Read the model definition and answer for the solid it produces. Units are mm, in the model's axes. Face numbers are marked on the shaded views. A direction names the side the tool comes from. Round coordinates to 2 decimals unless told otherwise and drop trailing zeros. Loops run counter-clockwise (first coordinate to the right, second up) from the corner with the lowest first, then second, coordinate; pieces in that order, holes last. Notation, with made-up numbers: (-30.5, 74.25) -> (23.5, 74.25) arc R24 cw to (23.5, 89.25) -> close; hole circle Ø1 at (29.5, 61.5). An arc over 180 degrees is marked (long way). Put each result on its own line as item: value.
from build123d import *

# Parameters (mm, degrees)
BOSS_EXTRUDE1_DEPTH = 5
SKETCH2_R           = 5
CUT_EXTRUDE1_DEPTH  = 3.5
SKETCH3_R           = 1
CUT_EXTRUDE2_DEPTH  = 2
CHAMFER3_SIZE       = 1.5


with BuildPart() as part:
    # Sketch1 → Boss-Extrude1 (new body)
    with BuildSketch(Plane.XY):
        with BuildLine():
            Line((0, -6.5), (13.5, -6.5))
            Line((13.5, -6.5), (13.5, 8.5))
            Line((13.5, 8.5), (11.5, 8.5))
            Line((11.5, 8.5), (-1.065452768, 6.412083156))
            ThreePointArc((-1.065452768, 6.412083156), (-6.477983502, -0.534536942), (0, -6.5))
        make_face()
    extrude(amount=BOSS_EXTRUDE1_DEPTH)

    # Sketch2 → Cut-Extrude1 (cut)
    with BuildSketch(Plane.XY.offset(5)):
        Circle(SKETCH2_R)
    extrude(amount=-CUT_EXTRUDE1_DEPTH, mode=Mode.SUBTRACT)

    # Sketch3 → Cut-Extrude2 (cut)
    with BuildSketch(Plane(origin=(13.5, 0, 0), x_dir=(0, 0, -1), z_dir=(1, 0, 0))):
        with Locations((-2.5, 6)):
            Circle(SKETCH3_R)
        with Locations(Location((-2.5, -4, 0), (0, 0, 180))):
            Circle(SKETCH3_R)
    extrude(amount=-CUT_EXTRUDE2_DEPTH, mode=Mode.SUBTRACT)

    # Chamfer3
    chamfer3_edges = [part.edges().sort_by_distance(p)[0] for p in [
        (5.217273616, 7.456041578, 0),
        (-6.477983502, -0.534536942, 0),
        (6.75, -6.5, 0),
    ]]
    chamfer(chamfer3_edges, length=CHAMFER3_SIZE)


solid = part.part
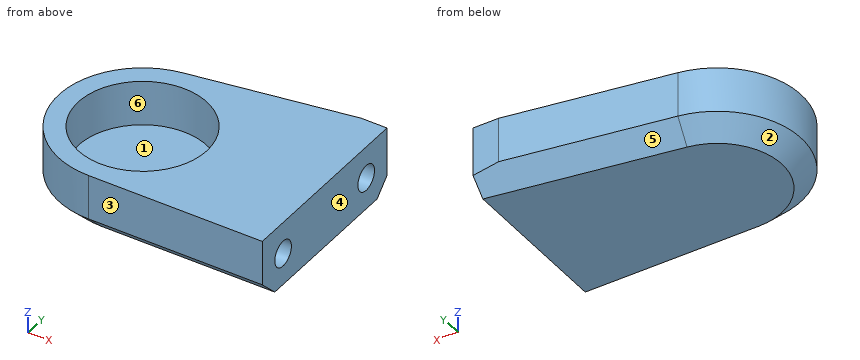
Item 1: The part is cut by section B-B (y = 0). Determine the outline of the cut face in (x, z), then the cut area to 3 significant figures.
Derived:
outline: (-6.5, 1.5) -> (-5, 0) -> (13.5, 0) -> (13.5, 5) -> (5, 5) -> (5, 1.5) -> (-5, 1.5) -> (-5, 5) -> (-6.5, 5) -> close
area: 63.9 mm^2
Item 2: The part is cut by section A-A (z = 2.5). Determine the outline of the cut face in (x, y).
Derived:
outline: (-1.07, 6.41) arc R6.5 ccw to (0, -6.5) -> (13.5, -6.5) -> (13.5, -5) -> (11.5, -5) -> (11.5, -3) -> (13.5, -3) -> (13.5, 5) -> (11.5, 5) -> (11.5, 7) -> (13.5, 7) -> (13.5, 8.5) -> (11.5, 8.5) -> close; hole circle Ø10 at (0, 0)
Item 3: The part is cut by section D-D (z = 3.9). Determine the outline of the cut face in (x, y).
Derived:
outline: (-1.07, 6.41) arc R6.5 ccw to (0, -6.5) -> (13.5, -6.5) -> (13.5, 8.5) -> (11.5, 8.5) -> close; hole circle Ø10 at (0, 0)
Item 4: Find the intervals of material crossed by line 1 along Y through (x, z) = (12, 2.5); line 2 along X through (y, z) = (-3.75, 1.25); line 3 along Y through (x, z) = (-4, 2.05), in increasing order.
Derived:
line 1: y = -6.5 to -5, -3 to 5, 7 to 8.5
line 2: x = -5 to 13.5
line 3: y = -5.12 to -3, 3 to 5.12
Item 5: For a pull along X with two mould halves and no side action, classify the marked faces 1, 2, 3 and 4 as pulls with the +X half, pulls with the -X half, needs draft (parallel to the pull), parting line crosses it, or undercut.
Derived:
face 1: undercut
face 2: pulls with the -X half
face 3: needs draft
face 4: pulls with the +X half
Item 6: Which of the six approach directions +Z, -Z, +X, -X, +Y, -Y give full straight-line access (tool end or side, diameter ignored) to the marked faces 5 and 6?
Derived:
face 5: -Z, -X, +Y
face 6: +Z
Item 7: The part is cut by section C-C (x = 12). Determine the outline of the cut face in (y, z).
Derived:
outline: (-6.5, 1.5) -> (-5, 0) -> (7.06, 0) -> (8.5, 1.42) -> (8.5, 5) -> (-6.5, 5) -> close; hole circle Ø2 at (-4, 2.5); hole circle Ø2 at (6, 2.5)
Item 8: Flat-ended cylindrical pins translate along their axes: pin 1 Ø2.5 at (y, z) = (6, 2.5) entering from -X; pin 2 Ø3 at (x, y) = (-2.5, 0.5) entering from +Z; pin 3 Ø1 at (y, z) = (-3.5, 1) entering from -X. Find the tip coordinate at first contact, or state that the pin passes through.
Derived:
pin 1: stops at x = -4.44
pin 2: stops at z = 1.5
pin 3: stops at x = -5.55
